```python
from build123d import *

# Parameters (mm, degrees)
SKETCH1_W           = 75
SKETCH1_H           = 30
BOSS_EXTRUDE1_DEPTH = 6
SKETCH2_W           = 4.5
SKETCH2_H           = 4.5
SKETCH2_W_2         = 38.5
SKETCH2_H_2         = 21
SKETCH2_W_3         = 5
SKETCH2_W_4         = 36
SKETCH2_W_5         = 6
SKETCH2_H_3         = 4
SKETCH2_H_4         = 8.5
BOSS_EXTRUDE4_DEPTH = 27
SKETCH7_W           = 4.5
SKETCH7_H           = 15
CUT_EXTRUDE1_DEPTH  = 6
SKETCH9_R           = 6.5
CUT_EXTRUDE2_DEPTH  = 30
SKETCH10_R          = 1.5
CUT_EXTRUDE3_DEPTH  = 50
SKETCH11_R          = 1.5
CUT_EXTRUDE4_DEPTH  = 10
SKETCH12_W          = 15
SKETCH12_H          = 26
CUT_EXTRUDE5_DEPTH  = 5


with BuildPart() as part:
    # Sketch1 → Boss-Extrude1 (new body)
    with BuildSketch(Plane.XZ.offset(4.342044015)):
        with Locations((-49.069594933, 13.200391181)):
            Rectangle(SKETCH1_W, SKETCH1_H)
    extrude(amount=BOSS_EXTRUDE1_DEPTH)

    # Sketch2 → Boss-Extrude4 (add)
    with BuildSketch(Plane(origin=(0, -10.342044015, 0), x_dir=(-1, 0, 0), z_dir=(0, -1, 0))):
        with Locations((84.319594933, -0.450391181)):
            Rectangle(SKETCH2_W, SKETCH2_H)
        with Locations((62.819594933, -0.450391181)):
            Rectangle(SKETCH2_W_2, SKETCH2_H)
        with Locations((84.319594933, -13.200391181)):
            Rectangle(SKETCH2_W, SKETCH2_H_2)
        with Locations((41.069594933, -0.450391181)):
            Rectangle(SKETCH2_W_3, SKETCH2_H)
        with Locations((84.319594933, -25.950391181)):
            Rectangle(SKETCH2_W, SKETCH2_H)
        with Locations((41.069594933, -4.950391181)):
            Rectangle(SKETCH2_W_3, SKETCH2_H)
        with Locations((64.069594933, -25.950391181)):
            Rectangle(SKETCH2_W_4, SKETCH2_H)
        with Locations((43.069594933, -25.950391181)):
            Rectangle(SKETCH2_W_5, SKETCH2_H)
        with Locations((43.069594933, -21.700391181)):
            Rectangle(SKETCH2_W_5, SKETCH2_H_3)
        with Locations((13.819594933, -23.950391181)):
            Rectangle(SKETCH2_W, SKETCH2_H_4)
    extrude(amount=BOSS_EXTRUDE4_DEPTH)

    # Sketch7 → Cut-Extrude1 (cut)
    with BuildSketch(Plane(origin=(-38.569594933, 0, 0), x_dir=(0, 0, -1), z_dir=(1, 0, 0))):
        with Locations((-4.950391181, -29.842044015)):
            Rectangle(SKETCH7_W, SKETCH7_H)
    extrude(amount=-CUT_EXTRUDE1_DEPTH, mode=Mode.SUBTRACT)

    # Sketch9 → Cut-Extrude2 (cut)
    with BuildSketch(Plane(origin=(0, -4.342044015, 0), x_dir=(1, 0, 0), z_dir=(0, 1, 0))):
        with Locations(Location((-70.319594933, -13.200391181, 0), (0, 0, 180))):
            Circle(SKETCH9_R)
    extrude(amount=-CUT_EXTRUDE2_DEPTH, mode=Mode.SUBTRACT)

    # Sketch10 → Cut-Extrude3 (cut)
    with BuildSketch(Plane.XY.offset(28.200391181)):
        with Locations((-77.569594933, -32.342044015)):
            Circle(SKETCH10_R)
    extrude(amount=-CUT_EXTRUDE3_DEPTH, mode=Mode.SUBTRACT)

    # Sketch11 → Cut-Extrude4 (cut)
    with BuildSketch(Plane.XY.offset(28.200391181)):
        with Locations((-54.569594933, -32.342044015)):
            Circle(SKETCH11_R)
    extrude(amount=-CUT_EXTRUDE4_DEPTH, mode=Mode.SUBTRACT)

    # Sketch12 → Cut-Extrude5 (cut)
    with BuildSketch(Plane.ZY.offset(86.569594933)):
        with Locations((13.200391181, -24.342044015)):
            Rectangle(SKETCH12_W, SKETCH12_H)
    extrude(amount=-CUT_EXTRUDE5_DEPTH, mode=Mode.SUBTRACT)


solid = part.part
```
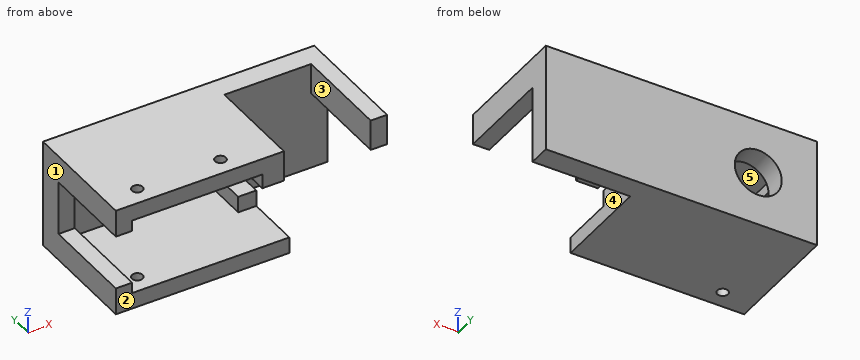
Work out the finished part from the listing and answer in its coordinate system (mm). Face numbers are marked on the shaded views. A direction names the side the tool comes from. Round coordinates to 2 decimals unless told otherwise and drop trailing zeros. Order: outer loops, then holes, each group sorted by start corner. A loop starts at its lowest first (then second) coordinate and runs counter-clockwise, first axis right, second up.
Q1. A tool of negligible diameter and unlimited length cuts with its end or side. For the marked faces 4 and 5, from which of +Z, -Z, +X, -X, +Y, -Y can it reach the whole face along a straight path? Write none if from no direction.
Solution:
face 4: +Z, -Z, +X, -Y
face 5: -Y
Q2. Given pin 1 Ø4 at (x, y) = (-77.57, -32.34) entering from +Z; pin 2 Ø4.5 at (y, z) = (-27.5, 1) entering from +X; pin 3 Ø9 at (x, z) = (-41.5, 11) entering from -Y; pin 4 Ø2.5 at (x, y) = (-54.57, -32.34) entering from +Z, each flat-ended and moving along its own axis, determine where each tip first touches the part or whether it passes through.
Solution:
pin 1: stops at z = 28.2
pin 2: stops at x = -38.57
pin 3: stops at y = -22.34
pin 4: stops at z = 2.7
Q3. The mould has two halves that part along X. Classify the marked faces 1, 2 and 3: pulls with the +X half, pulls with the -X half, needs draft (parallel to the pull), parting line crosses it, or undercut.
Solution:
face 1: pulls with the -X half
face 2: needs draft
face 3: undercut
Q4. Find the intervals of material crossed by line 1 along X through (y, z) = (-11.5, 23.5); line 2 along Z through (x, y) = (-80, -29); line 3 along X through (y, z) = (-15.5, 26), in increasing order.
Solution:
line 1: x = -86.57 to -82.07, -46.07 to -40.07, -16.07 to -11.57
line 2: z = -1.8 to 2.7, 23.7 to 28.2
line 3: x = -86.57 to -40.07, -16.07 to -11.57
Q5. A cutting plane is placed at D-D, the plane x = -52. Determine the outline of the cut face in (y, z).
Solution:
outline: (-37.34, -1.8) - (-4.34, -1.8) - (-4.34, 28.2) - (-37.34, 28.2) - (-37.34, 23.7) - (-10.34, 23.7) - (-10.34, 2.7) - (-37.34, 2.7) - close
Q6. A cutting plane is placed at C-C, the plane x = -78. Determine the outline of the cut face in (y, z).
Solution:
outline: (-37.34, -1.8) - (-33.78, -1.8) - (-33.78, 2.7) - (-37.34, 2.7) - close; (-37.34, 23.7) - (-33.78, 23.7) - (-33.78, 28.2) - (-37.34, 28.2) - close; (-30.91, -1.8) - (-4.34, -1.8) - (-4.34, 28.2) - (-30.91, 28.2) - (-30.91, 23.7) - (-10.34, 23.7) - (-10.34, 2.7) - (-30.91, 2.7) - close
Q7. A cutting plane is placed at B-B, the plane z = 17.5. Determine the outline of the cut face in (x, y).
Solution:
outline: (-86.57, -11.34) - (-82.07, -11.34) - (-82.07, -10.34) - (-75.19, -10.34) - (-75.19, -4.34) - (-86.57, -4.34) - close; (-65.44, -10.34) - (-11.57, -10.34) - (-11.57, -4.34) - (-65.44, -4.34) - close
Q8. A cutting plane is placed at A-A, the plane y = -17.5. Determine the outline of the cut face in (x, z).
Solution:
outline: (-86.57, -1.8) - (-38.57, -1.8) - (-38.57, 7.2) - (-43.57, 7.2) - (-43.57, 2.7) - (-82.07, 2.7) - (-82.07, 5.7) - (-86.57, 5.7) - close; (-86.57, 20.7) - (-82.07, 20.7) - (-82.07, 23.7) - (-46.07, 23.7) - (-46.07, 19.7) - (-40.07, 19.7) - (-40.07, 28.2) - (-86.57, 28.2) - close; (-16.07, 19.7) - (-11.57, 19.7) - (-11.57, 28.2) - (-16.07, 28.2) - close
